Geometry: final body of the model. Coordinates: model frame, mm. A direction names the side the tool comes from. Give positions to 0.01 mm unless a question says otherwise; leave off trailing zeros. Write each loop counter-clockwise with the first axis right and the second up, starting at its lowest first coordinate (ties: lowest second). Pieces come first, ordered by that corner, then holes. Notation, with made-up numbers: (46.25, 41.25) - (57.25, 41.25) arc R11 cw to (57.25, 61.25) - close; hole circle Ø3 at (41.25, 45). An arc over 180 degrees is marked (long way). Return JSON: item names as keys, results as strings.
Solid Edge part; units mm, degrees
sketch "Sketch1" plane through (0, 0, 0) normal (0, -1, 0) x (1, 0, 0)
  arc A0 (0, 7) -> (0, -7) centre (0, 0) cw
revolve "RevolvedProtrusion1" add sketch "Sketch1" angle 360 about axis through (0, 0, 7) along (0, 0, -1)
sketch "Sketch2" plane through (0, 0, 0) normal (1, 0, 0) x (0, 1, 0)
  circle A0 centre (0, 0) radius 4
extrude "Protrusion1" add sketch "Sketch2" along normal blind 9.8784
sketch "Sketch3" plane through (9.8784, 0, 0) normal (1, 0, 0) x (0, 1, 0)
  circle A0 centre (0, 0) radius 3
extrude "ExtrudedProtrusion_2" add sketch "Sketch3" along normal blind 10
cosmetic_thread "Thread1"
properties material "Steel"
Q1. Section query A-A, the plane z = 0. Return the cut outline in (x, y).
Answer key:
{"outline": "(5.74, -4) - (9.88, -4) - (9.88, -3) - (19.88, -3) - (19.88, 3) - (9.88, 3) - (9.88, 4) - (5.74, 4) arc R7 ccw (long way) to start"}
Q2. Material intervals for probe 1 along X at (y, z) = (4.75, 4.5); probe 2 along X at (y, z) = (5.5, -2); probe 3 along Z at (x, y) = (0.5, 1), sorted ascending. Write a range as [from, to].
Answer key:
{"probe 1": "x = [-2.49, 2.49]", "probe 2": "x = [-3.84, 3.84]", "probe 3": "z = [-6.91, 6.91]"}
Q3. Pin query (flat end, axial travel): P1, Ø4, axis at y = 5, z = 3.5, coming from the -X side; P2, Ø1, axis at x = -3, z = -5, coming from the +Y side; P3, Ø1, axis at y = 3.5, z = -0.5, coming from the -X side. Return the tip coordinate at first contact, or that it passes through.
Answer key:
{"P1": "stops at x = -5.67", "P2": "stops at y = 4.54", "P3": "stops at x = -6.31"}
Q4. Section query D-D, the plane z = 5. Return the cut outline in (x, y), plus the area to 3 significant figures.
Answer key:
{"outline": "circle Ø9.8 at (0, 0)", "area": "75.4 mm^2"}
Q5. Section query C-C, the plane x = -3. Return the cut outline in (y, z).
Answer key:
{"outline": "circle Ø12.65 at (0, 0)"}
Q6. Set-up query: faces 1 (the flat face through (19.878, 0, 0)), 2 (the cylindrical face through (15, -3, 0)). Return all of +Z, -Z, +X, -X, +Y, -Y with unobstructed straight access to the full face (end or side cutting, diameter ignored); none if empty.
Answer key:
{"face 1": "+Z, -Z, +X, +Y, -Y", "face 2": "+X"}
